from build123d import *

# Parameters (mm, degrees)
F1_DEPTH = 10
F0_W     = 10
F0_H     = 10
F2_DEPTH = 31.75


with BuildPart() as f1:
    # F0 (on Top) → F1 (new body)
    with BuildSketch(Plane.XY):
        Polygon((-17.5, -35), (0, -35), (0, 0), (-27.5, 0), (-27.5, -25), (-17.5, -25), align=None)
        Polygon((-27.5, 0), (0, 0), (0, 35), (-17.5, 35), (-17.5, 25), (-27.5, 25), align=None)
        Polygon((0, 0), (27.5, 0), (27.5, 25), (17.5, 25), (17.5, 35), (0, 35), align=None)
        Polygon((0, -35), (17.5, -35), (17.5, -25), (27.5, -25), (27.5, 0), (0, 0), align=None)
    extrude(amount=F1_DEPTH)

    # F0 (on Top) → F2 (join)
    with BuildSketch(Plane.XY):
        with Locations((22.5, 30)):
            Rectangle(F0_W, F0_H)
        with Locations((-22.5, 30)):
            Rectangle(F0_W, F0_H)
        with Locations((-22.5, -30)):
            Rectangle(F0_W, F0_H)
        with Locations((22.5, -30)):
            Rectangle(F0_W, F0_H)
    extrude(amount=F2_DEPTH)


solid = f1.part
Build history of the part. All positions in model axes, mm. A direction names the side the tool comes from. Give positions to 0.01 mm unless a question says otherwise; leave off trailing zeros. Loops run counter-clockwise (first coordinate to the right, second up) from the corner with the lowest first, then second, coordinate; pieces in that order, holes last. Notation, with made-up numbers: (-28.5, -37) - (12.5, -37) arc R32 cw to (12.5, -10) - close; hole circle Ø6 at (61.25, 34.5). An arc over 180 degrees is marked (long way). Write item = value, one per line. Start each with the question number.
1) Tool access for faces 5 (the flat face through (-17.5, 30, 21)), 6 (the flat face through (22, 25, 21)), 7 (the flat face through (22, 30, 31.75)): list every direction of +Z, -Z, +X, -X, +Y, -Y with a clear straight run to the whole face (end or side of a thin tool).
2) Band-saw the part on C-C on y = -8. Give the cut face in (x, z), plus the area to 3 significant figures.
3) Drop flat-ended pins along their axis: pin 1 Ø10 at (y, z) = (-19.5, 21.5) entering from -X; pin 2 Ø2 at (x, y) = (1, -7) entering from +Z. Give the stop position or say it passes through.
4) Band-saw the part on D-D on x = 8. Give the cut face in (y, z).
5) Band-saw the part on B-B on x = 20. Give the cut face in (y, z), plus the area to 4 significant figures.
6) Probe probe 1 along Y at (x, z) = (18, 10.5); probe 2 along X at (y, z) = (-32, 27); probe 3 along Z at (x, y) = (5.5, 7). List the from-to ranges inside material, lowest first. Write a range as from..to.
7) Band-saw the part on A-A on z = 21. Give the cut face in (x, y), plus the area to 3 significant figures.
8) Pull direction X, two halves, no side cores. Call faces 1 (the flat face through (27.5, 0, 9)), 2 (the flat face through (17.5, 30, 21)), 3 (the flat face through (0, 0, 0)), 4 (the flat face through (-27.5, 0, 9)): +X half, -X half, draft (parallel to the pull), parting line (faces both ways), or undercut.
Final values:
q1.face_5 = +Z, +Y, -Y
q1.face_6 = +Z, +X, -X
q1.face_7 = +Z, +X, -X, +Y, -Y
q2.outline = (-27.5, 0) - (27.5, 0) - (27.5, 10) - (-27.5, 10) - close
q2.area = 550 mm²
q3.pin_1 = through
q3.pin_2 = 10
q4.outline = (-35, 0) - (35, 0) - (35, 10) - (-35, 10) - close
q5.outline = (-35, 0) - (35, 0) - (35, 31.75) - (25, 31.75) - (25, 10) - (-25, 10) - (-25, 31.75) - (-35, 31.75) - close
q5.area = 1,135 mm²
q6.probe_1 = -35..-25, 25..35
q6.probe_2 = -27.5..-17.5, 17.5..27.5
q6.probe_3 = 0..10
q7.outline = (-27.5, -35) - (-17.5, -35) - (-17.5, -25) - (-27.5, -25) - close; (-27.5, 25) - (-17.5, 25) - (-17.5, 35) - (-27.5, 35) - close; (17.5, -35) - (27.5, -35) - (27.5, -25) - (17.5, -25) - close; (17.5, 25) - (27.5, 25) - (27.5, 35) - (17.5, 35) - close
q7.area = 400 mm²
q8.face_1 = +X half
q8.face_2 = undercut
q8.face_3 = draft
q8.face_4 = -X half
